Autodesk Inventor part; units mm, degrees
ref_plane "YZ Plane" through (0, 0, 0) normal (1, 0, 0) x (0, 1, 0)
ref_plane "XZ Plane" through (0, 0, 0) normal (0, 1, 0) x (-1, 0, 0)
ref_plane "XY Plane" through (0, 0, 0) normal (0, 0, 1) x (1, 0, 0)
sketch "Sketch1" plane through (0, 0, -15.875) normal (0, 0, 1) x (1, 0, 0)
  line L0 (-14.3205, -3.175) -> (14.3205, -3.175)
  arc A0 (14.3205, -3.175) -> (14.3205, 3.175) centre (14.3205, 0) ccw
  line L1 (14.3205, 3.175) -> (-14.3205, 3.175)
  arc A1 (-14.3205, 3.175) -> (-14.3205, -3.175) centre (-14.3205, 0) ccw
  line L2 (-14.3205, -3.175) -> (-14.3205, -3.175)
sketch "Sketch2" plane through (0, 0, -22.225) normal (0, 0, 1) x (1, 0, 0)
  line L0 (-25.4, -7.9375) -> (25.4, -7.9375)
  line L1 (25.4, -7.9375) -> (25.4, 7.9375)
  line L2 (25.4, 7.9375) -> (-25.4, 7.9375)
  line L3 (-25.4, 7.9375) -> (-25.4, -7.9375)
  line L4 (-25.4, -7.9375) -> (25.4, 7.9375) construction
  line L5 (25.4, -7.9375) -> (-25.4, 7.9375) construction
  point P0 (0, 0)
extrude "Extrusion1" add sketch "Sketch2" along normal blind 44.45
extrude "Extrusion2" cut sketch "Sketch1" along normal blind 31.75
properties part number "00000_Single_Mode_Rect"
Could you check a few things on this model? Use its own coordinates, in mm. A direction names the side the tool comes from. Round coordinates to 2 decimals unless told otherwise and drop trailing zeros. Loops run counter-clockwise (first coordinate to the right, second up) from the corner with the lowest first, then second, coordinate; pieces in that order, holes last.
Q1. Thinking about a two-plate mould opening in X: for faces 1 (the flat face through (0, 0, -15.875)), 2 (the flat face through (25.4, 0, 0)), 3 (the flat face through (0, -7.938, 0)), which applies, pulls with the +X half, pulls with the -X half, needs draft (parallel to the pull), parting line crosses it, or undercut?
Q2. Please list where these lines run through material, in increasing order: L1, parallel to Z at x = 1.5, y = 2 (3 decimals); L2, parallel to Y at x = 9, z = 6 (1 decimal); L3, parallel to X at y = -1, z = -10.
Q3. I want a section at B-B (x = -5). Write out the boundary of the cut face in (y, z) (1 decimal).
Q4. On a 3-axis mill with a long thin cutter (end or side, diameter ignored), from which of +Z, -Z, +X, -X, +Y, -Y can I reach the whole of each face in a straight line? I mean faces 4 (the flat face through (0, 0, 22.225)), 5 (the flat face through (0, -3.175, 0)). Say none if no direction works.
Answer below:
1. face 1: undercut
1. face 2: pulls with the +X half
1. face 3: needs draft
2. L1: z = -22.225 to -15.875, 15.875 to 22.225
2. L2: y = -7.9 to -3.2, 3.2 to 7.9
2. L3: x = -25.4 to -17.33, 17.33 to 25.4
3. outline: (-7.9, -22.2) - (7.9, -22.2) - (7.9, 22.2) - (-7.9, 22.2) - close; hole (-3.2, -15.9) - (3.2, -15.9) - (3.2, 15.9) - (-3.2, 15.9) - close
4. face 4: +Z, +X, -X, +Y, -Y
4. face 5: none
